Input: dimensioned drawing with shaded views. Units: mm. Origin: part minimum x, y, z. A direction names the side the tool comes from. Round coordinates to 2 decimals unless told otherwise and drop trailing zeros. Loops run counter-clockwise (first coordinate to the right, second up) from the corner with the lowest first, then second, coordinate; pieces in that order, holes last. Notation, with made-up numbers: (55.5, 20.5) -> (97.5, 20.5) arc R27 cw to (97.5, 53.5) -> close; hole circle Ø10 at (79.5, 49). An arc over 180 degrees is marked (long way). Answer as a JSON object with one key per item and string values.
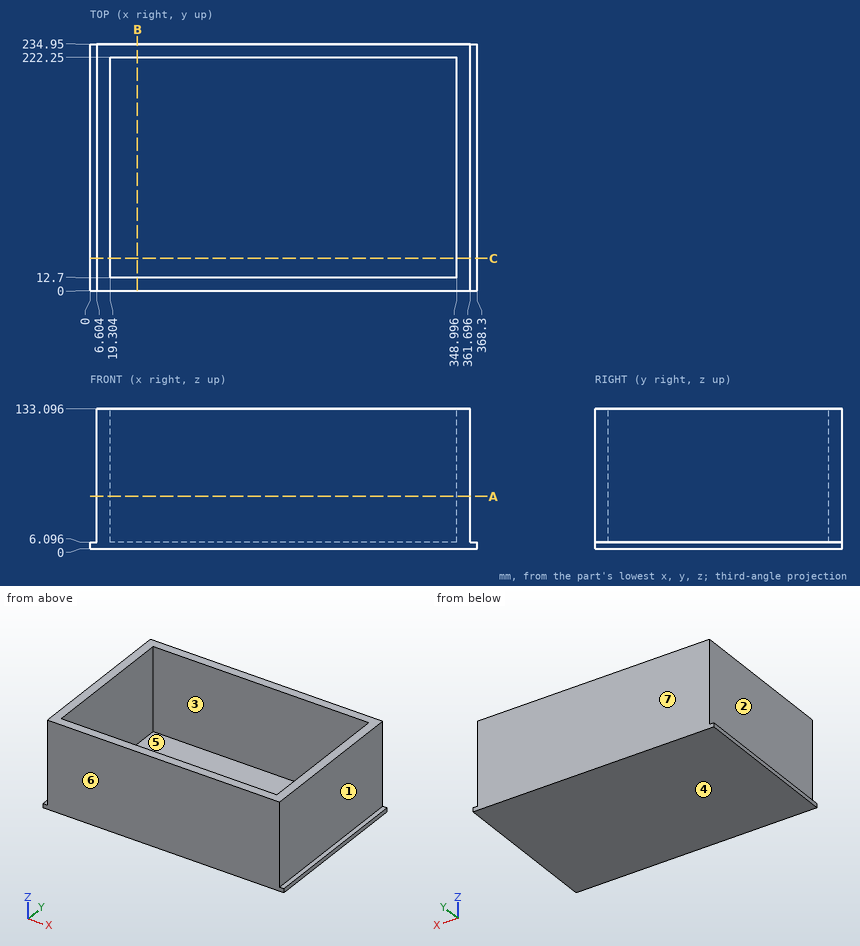
1) Section B-B, the plane x = 45. Output: boundary loops of the cut face in (y, z).
Output:
{"outline": "(0, 0) -> (234.95, 0) -> (234.95, 133.1) -> (222.25, 133.1) -> (222.25, 6.1) -> (12.7, 6.1) -> (12.7, 133.1) -> (0, 133.1) -> close"}
2) Ray query, probe 1 along X at (y, z) = (42, 43); probe 2 along Y at (x, z) = (46, 106); probe 3 along Z at (x, y) = (83, 215.5). Return the intervals inside material, ascending.
Output:
{"probe 1": "x = 6.6 to 19.3, 349 to 361.7", "probe 2": "y = 0 to 12.7, 222.25 to 234.95", "probe 3": "z = 0 to 6.1"}
3) Draft query along Y for the marked faces 5, 6 and 7. Return one class per face: +Y half, -Y half, draft (parallel to the pull), parting line (faces both ways), or undercut.
Output:
{"face 5": "undercut", "face 6": "-Y half", "face 7": "+Y half"}
4) Contact query for flat-ended pins moving along their axis: P1, Ø5.5, axis at x = 3, y = 146, coming from the +Z side; P2, Ø2, axis at y = 200, z = 106.5, coming from the +X side. Output: stop coordinate, or through.
Output:
{"P1": "stops at z = 6.1", "P2": "stops at x = 361.7"}
5) Section C-C, the plane y = 31. Output: boundary loops of the cut face in (x, z), plus the area to 3 significant figures.
Output:
{"outline": "(0, 0) -> (368.3, 0) -> (368.3, 6.1) -> (361.7, 6.1) -> (361.7, 133.1) -> (349, 133.1) -> (349, 6.1) -> (19.3, 6.1) -> (19.3, 133.1) -> (6.6, 133.1) -> (6.6, 6.1) -> (0, 6.1) -> close", "area": "5,470 mm^2"}
6) Section A-A, the plane z = 50. Output: boundary loops of the cut face in (x, y), plus the area to 3 significant figures.
Output:
{"outline": "(6.6, 0) -> (361.7, 0) -> (361.7, 234.95) -> (6.6, 234.95) -> close; hole (19.3, 12.7) -> (349, 12.7) -> (349, 222.25) -> (19.3, 222.25) -> close", "area": "14,300 mm^2"}
7) Reachability of the marked faces 1, 2, 3 and 4 from +Z, -Z, +X, -X, +Y, -Y: full face, straight path, thin tool, end or side. Return the list, or none.
Output:
{"face 1": "+Z, +X, +Y, -Y", "face 2": "+Z, -X, +Y, -Y", "face 3": "+Z", "face 4": "-Z, +X, -X, +Y, -Y"}
